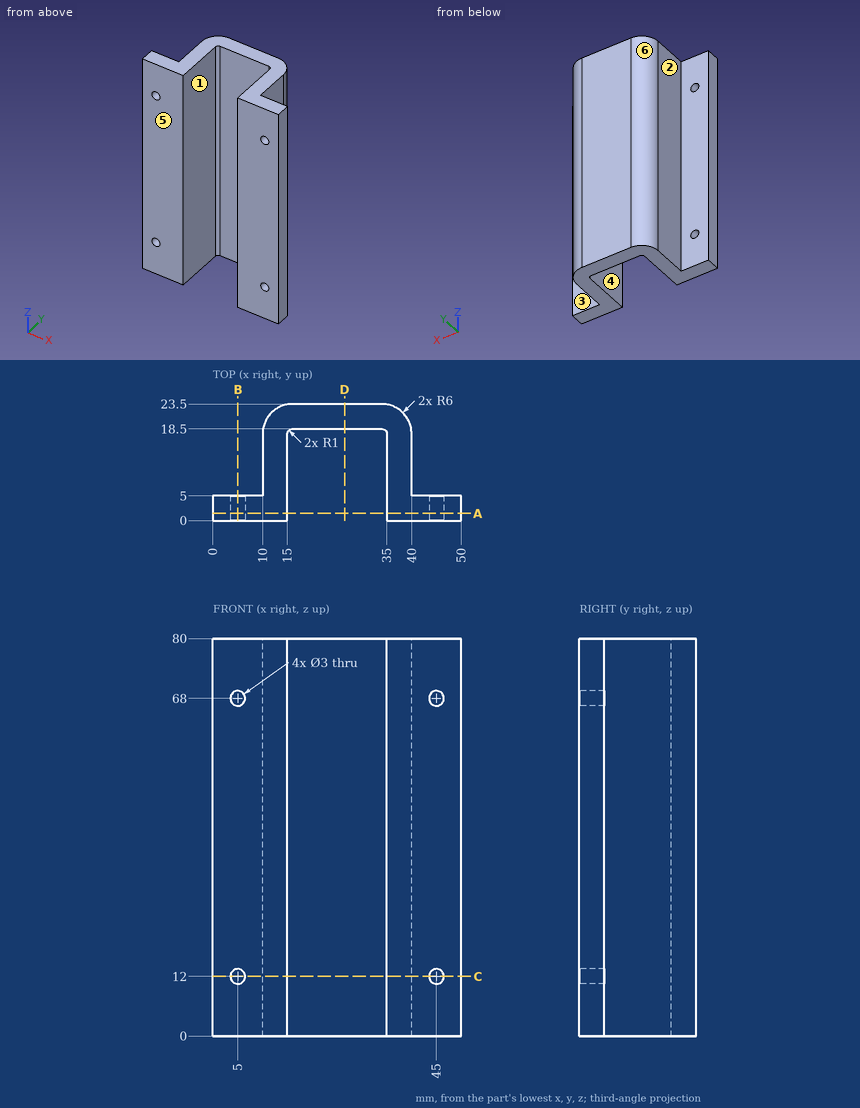
Part print with two shaded views. Sizes in mm from the minimum x, y, z corner. A direction names the side the tool comes from. Round coordinates to 2 decimals unless told otherwise and drop trailing zeros. Order: outer loops, then holes, each group sorted by start corner. A loop starts at its lowest first (then second) coordinate and runs counter-clockwise, first axis right, second up. Notation, with made-up numbers: (-14, 36.25) -> (5, 36.25) arc R21 cw to (5, 73.25) -> close; hole circle Ø9 at (-33, 33). An arc over 180 degrees is marked (long way). One line per question, with ' | ' between items.
Q1. Slice it at B-B (x = 5). Write the cut outline in (y, z).
Completed:
outline: (0, 0) -> (5, 0) -> (5, 10.5) -> (0, 10.5) -> close; (0, 13.5) -> (5, 13.5) -> (5, 66.5) -> (0, 66.5) -> close; (0, 69.5) -> (5, 69.5) -> (5, 80) -> (0, 80) -> close
Q2. Which spindle directions (+Z, -Z, +X, -X, +Y, -Y) get a long thin tool onto all of the face, cutting with end or side? Do the marked faces 1, 2 and 3. Say none if no direction does.
Completed:
face 1: +Z, -Z, -Y | face 2: +Z, -Z, -X, +Y | face 3: +Z, -Z, +X, +Y
Q3. Two-plate mould, pull along X, no slides. Class the marked faces 4, 5 and 6: released by +X, released by -X, zero draft, split by the parting line, or undercut.
Completed:
face 4: undercut | face 5: zero draft | face 6: released by -X
Q4. Slice it at A-A (y = 1.5). Write the cut outline in (x, z).
Completed:
outline: (0, 0) -> (15, 0) -> (15, 80) -> (0, 80) -> close; (35, 0) -> (50, 0) -> (50, 80) -> (35, 80) -> close; hole circle Ø3 at (5, 12); hole circle Ø3 at (5, 68); hole circle Ø3 at (45, 12); hole circle Ø3 at (45, 68)
Q5. Slice it at C-C (z = 12). Write the cut outline in (x, y), then the cut area to 3 significant figures.
Completed:
outline: (0, 0) -> (3.5, 0) -> (3.5, 5) -> (0, 5) -> close; (6.5, 0) -> (15, 0) -> (15, 17.5) arc R1 cw to (16, 18.5) -> (34, 18.5) arc R1 cw to (35, 17.5) -> (35, 0) -> (43.5, 0) -> (43.5, 5) -> (40, 5) -> (40, 17.5) arc R6 ccw to (34, 23.5) -> (16, 23.5) arc R6 ccw to (10, 17.5) -> (10, 5) -> (6.5, 5) -> close; (46.5, 0) -> (50, 0) -> (50, 5) -> (46.5, 5) -> close | area: 390 mm^2
Q6. Slice it at D-D (x = 26.5). Write the cut outline in (y, z).
Completed:
outline: (18.5, 0) -> (23.5, 0) -> (23.5, 80) -> (18.5, 80) -> close
Q7. Drop flat-ended pins along their axis: pin 1 (3.5 mm diameter, centred on x = 45, z = 68, fed in from +Y); pin 2 (14 mm diameter, centred on y = 12.5, z = 50, fed in from +X); pin 3 (2.5 mm diameter, centred on x = 5, z = 12, fed in from +Y); pin 4 (10 mm diameter, centred on y = 11.5, z = 30.5, fed in from -X). Give the stop position or say it passes through.
Completed:
pin 1: stops at y = 5 | pin 2: stops at x = 40 | pin 3: passes through | pin 4: stops at x = 10
Q8. Probe probe 1 along X at (y, z) = (2.9, 68); probe 2 along Z at (x, y) = (5, 1.1); probe 3 along X at (y, z) = (15.75, 50). List the from-to ranges inside material, lowest first.
Completed:
probe 1: x = 0 to 3.5, 6.5 to 15, 35 to 43.5, 46.5 to 50 | probe 2: z = 0 to 10.5, 13.5 to 66.5, 69.5 to 80 | probe 3: x = 10 to 15, 35 to 40
